Input: part model. Units: mm. Frame: model coordinates. A direction names the side the tool comes from. Give positions to 0.01 mm unless a question says otherwise; leave off trailing zeros. Loops run counter-clockwise (first coordinate to the right, second up) from the corner with the lowest first, then second, coordinate; pieces in that order, holes last.
from build123d import *

# Parameters (mm, degrees)
SM_BASE_FLANGE_1_DEPTH      = 40
SKETCH_6_R                  = 2.5
CUT_EXTRUDE_1_DEPTH         = 229.962879087
HOLE_WIZARD_M3_1_AT_2_COUNT = 2
HOLE_WIZARD_M3_1_AT_2_PITCH = 27
HOLE_WIZARD_M3_1_AT_3_COUNT = 2
HOLE_WIZARD_M3_1_AT_3_PITCH = 38.183766184
HOLE_WIZARD_M3_1_AT_4_COUNT = 2
HOLE_WIZARD_M3_1_AT_4_PITCH = 27
HOLE_WIZARD_M3_1_AT_5_COUNT = 2
HOLE_WIZARD_M3_1_AT_5_PITCH = 172.130764246
HOLE_WIZARD_M3_1_AT_6_COUNT = 2
HOLE_WIZARD_M3_1_AT_6_PITCH = 198.841645537
HOLE_WIZARD_M3_1_AT_7_COUNT = 2
HOLE_WIZARD_M3_1_AT_7_PITCH = 170
HOLE_WIZARD_M3_1_AT_8_COUNT = 2
HOLE_WIZARD_M3_1_AT_8_PITCH = 197
HOLE_WIZARD_7_0_7_1_D       = 7
HOLE_WIZARD_7_0_7_1_DEPTH   = 2
HOLE_WIZARD_7_0_7_1_TIP     = 2.103012167


# Sheet-metal steps are written as plain solids
with BuildPart() as part:
    # Sketch 1 → 基材-凸緣1 (new body)
    with BuildSketch(Plane.XY):
        with BuildLine():
            Line((0, 0), (38.083812051, 0))
            ThreePointArc((38.083812051, 0), (39.653461327, -0.494908516), (40.655374877, -1.800627676))
            Line((40.655374877, -1.800627676), (68.941214029, -79.515332038))
            ThreePointArc((68.941214029, -79.515332038), (69.210895211, -79.866787396), (69.633391614, -80))
            Line((69.633391614, -80), (148.548612075, -80))
            ThreePointArc((148.548612075, -80), (148.998913005, -79.84633107), (149.261331062, -79.44944087))
            Line((149.261331062, -79.44944087), (169.46608317, -2.045425081))
            ThreePointArc((169.46608317, -2.045425081), (170.441012922, -0.570907404), (172.11396096, 0))
            Line((172.11396096, 0), (210, 0))
            Line((210, 0), (210, -2))
            Line((210, -2), (172.11396096, -2))
            ThreePointArc((172.11396096, -2), (171.66366003, -2.15366893), (171.401241973, -2.55055913))
            Line((171.401241973, -2.55055913), (151.196489865, -79.954574919))
            ThreePointArc((151.196489865, -79.954574919), (150.221560113, -81.429092596), (148.548612075, -82))
            Line((148.548612075, -82), (69.633391614, -82))
            ThreePointArc((69.633391614, -82), (68.063742338, -81.505091484), (67.061828788, -80.199372324))
            Line((67.061828788, -80.199372324), (38.775989635, -2.484667962))
            ThreePointArc((38.775989635, -2.484667962), (38.506308454, -2.133212604), (38.083812051, -2))
            Line((38.083812051, -2), (0, -2))
            Line((0, -2), (0, 0))
        make_face()
    extrude(amount=SM_BASE_FLANGE_1_DEPTH)

    # 草圖6 → 除料-伸長1 (cut, through all)
    with BuildSketch(Plane.XZ.offset(82)):
        with Locations((137.091001844, 20)):
            Circle(SKETCH_6_R)
        with Locations((81.091001844, 20)):
            Circle(SKETCH_6_R)
    extrude(amount=-CUT_EXTRUDE_1_DEPTH, mode=Mode.SUBTRACT)

    # 草圖13 → M3 高錐坑頭螺釘的錐孔1 (revolve, cut)
    with BuildSketch(Plane(origin=(6.5, -2, 33.5), x_dir=(0, 0, -1), z_dir=(1, 0, 0))):
        Polygon((0, 0), (0, 3.021463052), (1.7, 2), (1.7, 1.45), (3.15, 0), align=None)
    hole_wizard_m3_1 = revolve(axis=Axis((6.5, -8.35, 33.5), (0, 1, 0)), mode=Mode.SUBTRACT)

    # M3 高錐坑頭螺釘的錐孔1 at 2: M3 高錐坑頭螺釘的錐孔1 ×2
    with Locations(*[(i * HOLE_WIZARD_M3_1_AT_2_PITCH, 0, 0) for i in range(1, HOLE_WIZARD_M3_1_AT_2_COUNT)]):
        add(hole_wizard_m3_1, mode=Mode.SUBTRACT)

    # M3 高錐坑頭螺釘的錐孔1 at 3: M3 高錐坑頭螺釘的錐孔1 ×2
    with Locations(*[Vector(0.7071067811865476, 0, -0.7071067811865476) * (i * HOLE_WIZARD_M3_1_AT_3_PITCH) for i in range(1, HOLE_WIZARD_M3_1_AT_3_COUNT)]):
        add(hole_wizard_m3_1, mode=Mode.SUBTRACT)

    # M3 高錐坑頭螺釘的錐孔1 at 4: M3 高錐坑頭螺釘的錐孔1 ×2
    with Locations(*[(0, 0, -i * HOLE_WIZARD_M3_1_AT_4_PITCH) for i in range(1, HOLE_WIZARD_M3_1_AT_4_COUNT)]):
        add(hole_wizard_m3_1, mode=Mode.SUBTRACT)

    # M3 高錐坑頭螺釘的錐孔1 at 5: M3 高錐坑頭螺釘的錐孔1 ×2
    with Locations(*[Vector(0.9876212468143859, 0, -0.15685749214110833) * (i * HOLE_WIZARD_M3_1_AT_5_PITCH) for i in range(1, HOLE_WIZARD_M3_1_AT_5_COUNT)]):
        add(hole_wizard_m3_1, mode=Mode.SUBTRACT)

    # M3 高錐坑頭螺釘的錐孔1 at 6: M3 高錐坑頭螺釘的錐孔1 ×2
    with Locations(*[Vector(0.9907381296691129, 0, -0.13578644416784796) * (i * HOLE_WIZARD_M3_1_AT_6_PITCH) for i in range(1, HOLE_WIZARD_M3_1_AT_6_COUNT)]):
        add(hole_wizard_m3_1, mode=Mode.SUBTRACT)

    # M3 高錐坑頭螺釘的錐孔1 at 7: M3 高錐坑頭螺釘的錐孔1 ×2
    with Locations(*[(i * HOLE_WIZARD_M3_1_AT_7_PITCH, 0, 0) for i in range(1, HOLE_WIZARD_M3_1_AT_7_COUNT)]):
        add(hole_wizard_m3_1, mode=Mode.SUBTRACT)

    # M3 高錐坑頭螺釘的錐孔1 at 8: M3 高錐坑頭螺釘的錐孔1 ×2
    with Locations(*[(i * HOLE_WIZARD_M3_1_AT_8_PITCH, 0, 0) for i in range(1, HOLE_WIZARD_M3_1_AT_8_COUNT)]):
        add(hole_wizard_m3_1, mode=Mode.SUBTRACT)

    # Ø7.0 (7) 直徑孔1
    with Locations(Plane(origin=(0, -2, 0), x_dir=(-1, 0, 0), z_dir=(0, -1, 0))):
        with Locations((-20, -20), (-190, -20)):
            Hole(HOLE_WIZARD_7_0_7_1_D / 2, depth=HOLE_WIZARD_7_0_7_1_DEPTH)
            with Locations((0, 0, -(HOLE_WIZARD_7_0_7_1_DEPTH + HOLE_WIZARD_7_0_7_1_TIP / 2))):  # 118° drill point
                Cone(0, HOLE_WIZARD_7_0_7_1_D / 2, HOLE_WIZARD_7_0_7_1_TIP, mode=Mode.SUBTRACT)


solid = part.part
(1) Cut plane A-A (x = 190). Return the cut outline in (y, z), and give its area (3 significant figures).
Values follow:
outline: (-2, 0) - (0, 0) - (0, 16.5) - (-2, 16.5) - close; (-2, 23.5) - (0, 23.5) - (0, 40) - (-2, 40) - close
area: 66.0 mm2
(2) Cut plane B-B (z = 26.5). Return the cut outline in (x, y), and give its area (3 significant figures).
Values follow:
outline: (0, -2) - (38.08, -2) arc R0.74 cw to (38.78, -2.48) - (67.06, -80.2) arc R2.74 ccw to (69.63, -82) - (148.55, -82) arc R2.74 ccw to (151.2, -79.95) - (171.4, -2.55) arc R0.74 cw to (172.11, -2) - (210, -2) - (210, 0) - (172.11, 0) arc R2.74 ccw to (169.47, -2.05) - (149.26, -79.45) arc R0.74 cw to (148.55, -80) - (69.63, -80) arc R0.74 cw to (68.94, -79.52) - (40.66, -1.8) arc R2.74 ccw to (38.08, 0) - (0, 0) - close
area: 653 mm2
(3) Reachability of faces 4 (the cylindrical face through (193.34, -0.99, 18.95)), 5 (the flat face through (159.222, -41.289, 19.72)), 6 (the flat face through (196, -2, 20)), 7 (the flat face through (15, -2, 20)) from +Z, -Z, +X, -X, +Y, -Y: full face, straight path, thin tool, end or side. Return the list, or none.
Values follow:
face 4: +Y, -Y
face 5: +Z, -Z, +Y
face 6: +Z, -Z, +X, -Y
face 7: +Z, -Z, -X, -Y
(4) Cut plane D-D (x = 127). Return the cut outline in (y, z).
Values follow:
outline: (-82, 0) - (-80, 0) - (-80, 40) - (-82, 40) - close
(5) Pin query (flat end, axial travel): pin 1 Ø1.5 at (y, z) = (-22.5, 13.5) entering from +X; pin 2 Ø4 at (x, z) = (65.5, 12) entering from -Y; pin 3 Ø12 at (y, z) = (-55, 19.5) entering from -X. Return the tip coordinate at first contact, or that it passes through.
Values follow:
pin 1: stops at x = 166.39
pin 2: stops at y = -80.98
pin 3: stops at x = 55.71
(6) Cut plane C-C (y = -4.5). Return the cut outline in (x, z).
Values follow:
outline: (39.51, 0) - (41.64, 0) - (41.64, 40) - (39.51, 40) - close; (168.83, 0) - (170.89, 0) - (170.89, 40) - (168.83, 40) - close
(7) Mould query, pull axis Z, two halves, no side actions, for faces 1 (the flat face through (105.5, -80.3, 40)), 2 (the flat face through (109, -80, 20)), 3 (the cylindrical face through (21.88, -0.99, 17.05)). Classes: +Z half, -Z half, draft (parallel to the pull), parting line (faces both ways), or undercut.
Values follow:
face 1: +Z half
face 2: draft
face 3: undercut
(8) Ray query, probe 1 along Z at (x, y) = (33.5, -0.35); probe 2 along Y at (x, z) = (118, 9); probe 3 along X at (y, z) = (-60.5, 24). Return the intervals inside material, ascending.
Values follow:
probe 1: z = 0 to 4.8, 8.2 to 31.8, 35.2 to 40
probe 2: y = -82 to -80
probe 3: x = 59.89 to 62.02, 154.21 to 156.27
